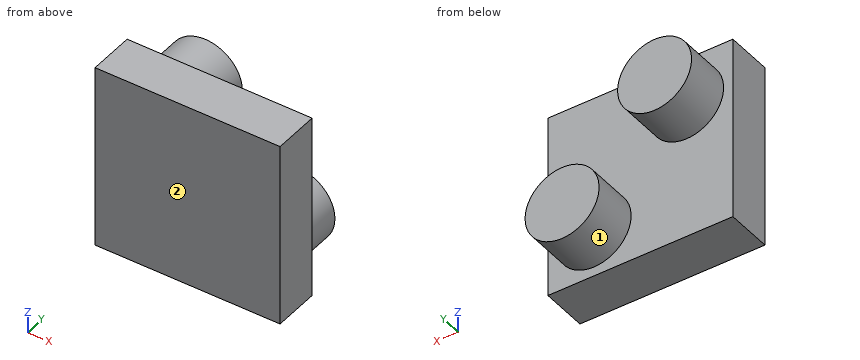
from build123d import *

# Parameters (mm, degrees)
SKETCH1_W           = 10
SKETCH1_H           = 10
BOSS_EXTRUDE1_DEPTH = 5
SKETCH2_W           = 10
SKETCH2_H           = 10
SKETCH2_R           = 2
CUT_EXTRUDE1_DEPTH  = 2.5


with BuildPart() as part:
    # Sketch1 → Boss-Extrude1 (new body)
    with BuildSketch(Plane(origin=(0, 0, 0), x_dir=(1, 0, 0), z_dir=(0, 1, 0))):
        Rectangle(SKETCH1_W, SKETCH1_H)
    extrude(amount=BOSS_EXTRUDE1_DEPTH)

    # Sketch2 → Cut-Extrude1 (cut)
    with BuildSketch(Plane(origin=(0, 5, 0), x_dir=(1, 0, 0), z_dir=(0, 1, 0))):
        Rectangle(SKETCH2_W, SKETCH2_H)
        with Locations((-2.5, -2.5)):
            Circle(SKETCH2_R, mode=Mode.SUBTRACT)
        with Locations((2.5, 2.5)):
            Circle(SKETCH2_R, mode=Mode.SUBTRACT)
    extrude(amount=-CUT_EXTRUDE1_DEPTH, mode=Mode.SUBTRACT)


solid = part.part
The model under review builds one solid part; all positions refer to its coordinate system, in mm. Face numbers are marked on the shaded views. A direction names the side the tool comes from. Round coordinates to 2 decimals unless told otherwise and drop trailing zeros. Write each loop counter-clockwise with the first axis right and the second up, starting at its lowest first coordinate (ties: lowest second). Pieces come first, ordered by that corner, then holes. Notation, with made-up numbers: (23, -6.5) - (59, -6.5) arc R32 ccw to (59, 28.5) - close; hole circle Ø9 at (44.5, -21). An arc over 180 degrees is marked (long way). One line per item, written item: value. Start each with the question number.
1. Consider section B-B on z = -2.5. Write out the cut boundary in (x, y), and give its area (3 significant figures).
2. Machinability: for the marked faces 1 and 2, which of the approach directions +Z, -Z, +X, -X, +Y, -Y give a long, thin tool a straight path to every point of the face, cutting with its end or side? Answer none if there is none.
3. Consider section D-D on z = 0. Write out the cut boundary in (x, y).
4. Consider section C-C on y = 3.1. Write out the cut boundary in (x, z), and give its area (3 significant figures).
5. To check wall thickness, follow L1, parallel to Y at x = 2, z = 0.5; L2, parallel to X at y = 4.85, z = 1.75; L3, parallel to Z at x = 4, y = 4.75. State the ranges of each line that lie inside material, in increasing order. Write a range as from..to.
6. Clearance check with flat-ended pins moving along their axes: P1, Ø1, axis at x = 2.5, y = 4, coming from the -Z side; P2, Ø4, axis at x = -1, z = -3.5, coming from the -Y side. State where each tip first meets the part, or that it passes through.
7. Consider section A-A on x = 2.5. Write out the cut boundary in (y, z).
Checks:
1. outline: (-5, 0) - (5, 0) - (5, 2.5) - (4.5, 2.5) - (4.5, 5) - (0.5, 5) - (0.5, 2.5) - (-5, 2.5) - close
1. area: 35.0 mm^2
2. face 1: +Y
2. face 2: +Z, -Z, +X, -X, -Y
3. outline: (-5, 0) - (5, 0) - (5, 2.5) - (-5, 2.5) - close
4. outline: circle Ø4 at (-2.5, 2.5); circle Ø4 at (2.5, -2.5)
4. area: 25.1 mm^2
5. L1: y = 0..2.5
5. L2: x = -4.35..-0.65
5. L3: z = -3.82..-1.18
6. P1: stops at z = -4.5
6. P2: stops at y = 0
7. outline: (0, -5) - (2.5, -5) - (2.5, -4.5) - (5, -4.5) - (5, -0.5) - (2.5, -0.5) - (2.5, 5) - (0, 5) - close
